Input: part model. Units: mm. Frame: model coordinates. Face numbers are marked on the shaded views. Round coordinates to 2 decimals unless told otherwise and drop trailing zeros. Order: outer loops, then holes, each group sorted by start corner. A loop starts at its lowest first (then second) coordinate and runs counter-clockwise, first axis right, second up.
Item 1: Cut plane D-D on x = -18. Output: boundary loops of the cut face in (y, z), then the cut area to 3 significant figures.
Item 2: First-contact query: pin 1 (1.5 mm diameter, centred on x = -2, z = -44, fed in from -Y); pin 2 (12 mm diameter, centred on x = -17, z = -25.5, fed in from +Y); pin 3 (1 mm diameter, centred on x = 9, z = -21, fed in from -Y). Flat tips, straight axial feed; report the tip coordinate or a pass-through.
Item 3: Mould query, pull axis Z, two halves, no side actions, for the marked faces 1 and 2. Classes: released by +Z, released by -Z, zero draft, split by the parting line, or undercut.
Item 4: Line query: L1, parallel to Y at x = 0, z = -24; L2, parallel to Z at x = 17, y = -5.5; L3, parallel to Y at x = -24.5, z = -0.5. Output: solid intervals per line, ascending.
Item 5: Cut plane C-C on x = -9.5. Output: boundary loops of the cut face in (y, z), then the cut area to 3 significant figures.
Item 6: Cut plane A-A on y = -1.5. Output: boundary loops of the cut face in (x, z).
Item 7: Cut plane B-B on z = -15. Output: boundary loops of the cut face in (x, y) (3 decimals).
```python
from build123d import *

# Parameters (mm, degrees)
F1_DEPTH = 12.7
F2_SIZE2 = 12.69999
F2_SIZE  = 12.69999


# Not quite as in the source:
# - a fillet or chamfer is up to 0.001 mm smaller than in the source, because OpenCascade refuses the exact size


with BuildPart() as f1:
    # F0 (on Top) → F1 (new body)
    with BuildSketch(Plane.XY):
        Polygon((-31.75, 13.1512806053), (-31.75, -13.1512806053), (-13.1512806053, -31.75), (13.1512806053, -31.75), (31.75, -13.1512806053), (31.75, 13.1512806053), (13.1512806053, 31.75), (-13.1512806053, 31.75), align=None)
    extrude(amount=F1_DEPTH)

    # F2 (size 12.7 and 12.7 in the source; OpenCascade refuses exactly that, so slightly less here)
    f2_edges = [f1.edges().sort_by_distance(p)[0] for p in [
        (-22.45064, 22.45064, 12.7),
        (-31.75, 0, 12.7),
        (-22.45064, -22.45064, 12.7),
        (0, -31.75, 12.7),
        (22.45064, -22.45064, 12.7),
        (31.75, 0, 12.7),
        (22.45064, 22.45064, 12.7),
        (0, 31.75, 12.7),
    ]]
    chamfer(f2_edges, length=F2_SIZE, length2=F2_SIZE2)

    # F1_face (on face) → F5 section 0
    with BuildSketch(Plane(origin=(0, 0, 0), x_dir=(1, 0, 0), z_dir=(0, 0, -1)), mode=Mode.PRIVATE) as f5_s0:
        Polygon((-31.75, -13.1512806053), (-13.1512806053, -31.75), (13.1512806053, -31.75), (31.75, -13.1512806053), (31.75, 13.1512806053), (13.1512806053, 31.75), (-13.1512806053, 31.75), (-31.75, 13.1512806053), align=None)
    loft([f5_s0.sketch, Vertex(0, 0, -50.8)])


solid = f1.part
```
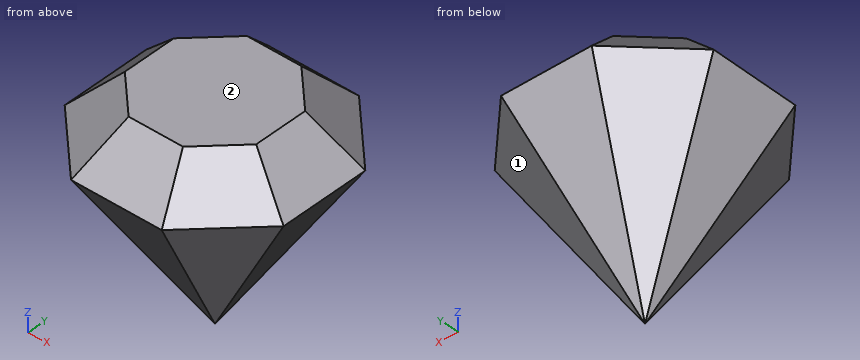
From the geometry:
1. outline: (-26.9, 0) - (-7.46, -22) - (7.46, -22) - (26.9, 0) - (8.94, 12.7) - (-8.94, 12.7) - close
1. area: 1,210 mm2
2. pin 1: stops at y = -4.72
2. pin 2: stops at y = 13.37
2. pin 3: stops at y = -18.01
3. face 1: released by -Z
3. face 2: released by +Z
4. L1: y = -16.75 to 16.75
4. L2: z = -23.6 to 12.7
4. L3: y = -19.96 to 19.96
5. outline: (-31.75, 0) - (-22.94, -14.1) - (-3.94, -35.6) - (3.94, -35.6) - (22.94, -14.1) - (31.75, 0) - (22.94, 8.81) - (17.44, 12.7) - (-17.44, 12.7) - (-22.94, 8.81) - close
5. area: 1,990 mm2
6. outline: (-31.75, 0) - (-3.62, -45.01) - (-0.62, -48.4) - (0.62, -48.4) - (3.62, -45.01) - (31.75, 0) - (19.05, 12.7) - (-19.05, 12.7) - close
7. outline: (-22.375, -9.268) - (-9.268, -22.375) - (9.268, -22.375) - (22.375, -9.268) - (22.375, 9.268) - (9.268, 22.375) - (-9.268, 22.375) - (-22.375, 9.268) - close
